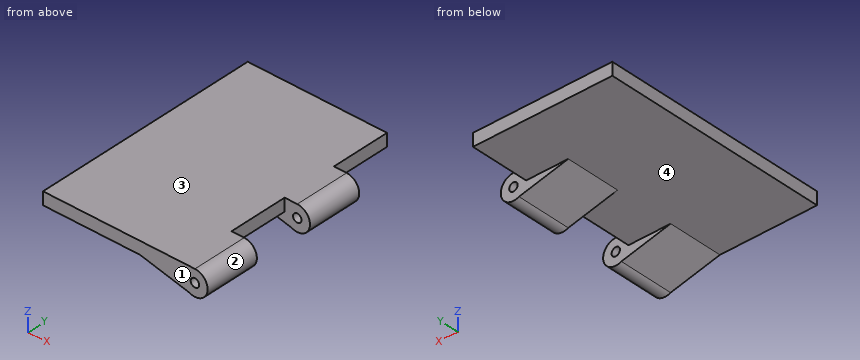
```python
from build123d import *

# Parameters (mm, degrees)
BOSS_EXTRUDE1_DEPTH = 6.5
SKETCH2_W           = 15
SKETCH2_H           = 1.5
BOSS_EXTRUDE2_DEPTH = 7
BOSS_EXTRUDE3_DEPTH = 6.5
SKETCH4_W           = 15
SKETCH4_H           = 1.5
BOSS_EXTRUDE4_DEPTH = 7
SKETCH5_R           = 0.5
CUT_EXTRUDE1_DEPTH  = 27
SKETCH6_W           = 1.5
SKETCH6_H           = 27
BOSS_EXTRUDE5_DEPTH = 1.5


with BuildPart() as part:
    # Sketch1 → Boss-Extrude1 (new body)
    with BuildSketch(Plane(origin=(0, 0, 0), x_dir=(1, 0, 0), z_dir=(0, 1, 0))):
        with BuildLine():
            Line((-7.5, -0.75), (9, -0.75))
            ThreePointArc((9, -0.75), (10.461586794, 1.08728926), (8.342696629, 2.098314607))
            Line((8.342696629, 2.098314607), (2.5, 0.75))
            Line((2.5, 0.75), (-7.5, 0.75))
            Line((-7.5, 0.75), (-7.5, -0.75))
        make_face()
    extrude(amount=BOSS_EXTRUDE1_DEPTH)

    # Sketch2 → Boss-Extrude2 (add)
    with BuildSketch(Plane(origin=(0, 6.5, 0), x_dir=(1, 0, 0), z_dir=(0, 1, 0))):
        Rectangle(SKETCH2_W, SKETCH2_H)
    extrude(amount=BOSS_EXTRUDE2_DEPTH)

    # Sketch3 → Boss-Extrude3 (add)
    with BuildSketch(Plane(origin=(0, 13.5, 0), x_dir=(1, 0, 0), z_dir=(0, 1, 0))):
        with BuildLine():
            Line((-7.5, -0.75), (9, -0.75))
            ThreePointArc((9, -0.75), (10.461586794, 1.08728926), (8.342696629, 2.098314607))
            Line((8.342696629, 2.098314607), (2.5, 0.75))
            Line((2.5, 0.75), (-7.5, 0.75))
            Line((-7.5, 0.75), (-7.5, -0.75))
        make_face()
    extrude(amount=BOSS_EXTRUDE3_DEPTH)

    # Sketch4 → Boss-Extrude4 (add)
    with BuildSketch(Plane(origin=(0, 20, 0), x_dir=(1, 0, 0), z_dir=(0, 1, 0))):
        Rectangle(SKETCH4_W, SKETCH4_H)
    extrude(amount=BOSS_EXTRUDE4_DEPTH)

    # Sketch5 → Cut-Extrude1 (cut)
    with BuildSketch(Plane.XZ):
        with Locations(Location((9, -0.75, 0), (0, 0, 90))):
            Circle(SKETCH5_R)
    extrude(amount=-CUT_EXTRUDE1_DEPTH, mode=Mode.SUBTRACT)

    # Sketch6 → Boss-Extrude5 (add)
    with BuildSketch(Plane.ZY.offset(7.5)):
        with Locations((0, 13.5)):
            Rectangle(SKETCH6_W, SKETCH6_H)
    extrude(amount=BOSS_EXTRUDE5_DEPTH)


solid = part.part
```
Could you check a few things on this model? Use its own coordinates, in mm. Face numbers are marked on the shaded views. A direction names the side the tool comes from. Round coordinates to 2 decimals unless told otherwise and drop trailing zeros. Write each loop counter-clockwise with the first axis right and the second up, starting at its lowest first coordinate (ties: lowest second). Pieces come first, ordered by that corner, then holes.
(1) For pin 1 (8 mm diameter, centred on x = 1.5, y = 12.5, fed in from -Z); pin 2 (0.8 mm diameter, centred on y = 11.5, z = 0, fed in from +X), each with a flat end and sliding along its axis, tell me the tip position at first contact or that it passes through.
Findings below:
pin 1: stops at z = -1.41
pin 2: stops at x = 7.5
(2) If I drill on probe 1 along Y at (x, z) = (8.25, -1.6); probe 2 along Z at (x, y) = (9, 1.5); probe 3 along Z at (x, y) = (0.25, 6.75), over which ranges is the centre line in solid material (lowest first)?
Findings below:
probe 1: y = 0 to 6.5, 13.5 to 20
probe 2: z = -2.25 to -1.25, -0.25 to 0.75
probe 3: z = -0.75 to 0.75
(3) Which directions (+Z, -Z, +X, -X, +Y, -Y) give clear straight access to the entire face, cutting with the end or side of a thin tool? Please do the marked faces 3 and 4.
Findings below:
face 3: +Z, +X, -X, +Y, -Y
face 4: -Z, -X
(4) Thinking about a two-plate mould opening in Y: for the marked faces 1 and 2, which applies, +Y half, -Y half, draft (parallel to the pull), parting line (faces both ways), or undercut?
Findings below:
face 1: -Y half
face 2: draft
(5) Suppose I cut it at B-B on y = 19.25. Write out the boundary of the cut face in (x, z), and give its area (3 significant figures).
Findings below:
outline: (-9, -0.75) - (2.5, -0.75) - (8.34, -2.1) arc R1.5 ccw (long way) to (9, 0.75) - (-9, 0.75) - close; hole circle Ø1 at (9, -0.75)
area: 34.6 mm2
(6) Suppose I cut it at D-D on z = 0.1. Write out the boundary of the cut face in (x, y).
Findings below:
outline: (-9, 0) - (10.24, 0) - (10.24, 6.5) - (7.5, 6.5) - (7.5, 13.5) - (10.24, 13.5) - (10.24, 20) - (7.5, 20) - (7.5, 27) - (-9, 27) - close
(7) Suppose I cut it at C-C on x = -1.5. Write out the boundary of the cut face in (y, z), and give its area (3 significant figures).
Findings below:
outline: (0, -0.75) - (27, -0.75) - (27, 0.75) - (0, 0.75) - close
area: 40.5 mm2
(8) Suppose I cut it at A-A on z = -1.65. Write out the boundary of the cut face in (x, y), and give its area (3 significant figures).
Findings below:
outline: (6.4, 0) - (10.2, 0) - (10.2, 6.5) - (6.4, 6.5) - close; (6.4, 13.5) - (10.2, 13.5) - (10.2, 20) - (6.4, 20) - close
area: 49.4 mm2
